from build123d import *

# Parameters (mm, degrees)
SKETCH1_R           = 2.5
SKETCH1_W           = 50
SKETCH1_H           = 22.5
BOSS_EXTRUDE1_DEPTH = 3


with BuildPart() as part:
    # Sketch1 → Boss-Extrude1 (new body)
    # profile 1 of 7: a face of its own
    with BuildSketch(Plane.XY):
        with BuildLine():
            ThreePointArc((22.5, 0), (15.909902577, 15.909902577), (0, 22.5))
            Line((0, 22.5), (-22.5, 0))
            ThreePointArc((-22.5, 0), (-22.471786645, -1.126412439), (-22.387217335, -2.25))
            ThreePointArc((-22.387217335, -2.25), (1.126412439, -22.471786645), (22.5, 0))
        make_face()
        with BuildLine():
            ThreePointArc((-7.5, 5), (-9.267766953, 9.267766953), (-5, 7.5))
            Line((-5, 7.5), (-5, 9))
            Line((-5, 9), (-2.405779746, 18.179870439))
            ThreePointArc((-2.405779746, 18.179870439), (0, 20), (2.405779746, 18.179870439))
            Line((2.405779746, 18.179870439), (5, 9))
            Line((5, 9), (5, 7.5))
            ThreePointArc((5, 7.5), (7.5, 10), (10, 7.5))
            ThreePointArc((10, 7.5), (9.267766953, 5.732233047), (7.5, 5))
            Line((7.5, 5), (9, 5))
            Line((9, 5), (18.179870439, 2.405779746))
            ThreePointArc((18.179870439, 2.405779746), (19.493699588, 1.508363998), (20, 0))
            ThreePointArc((20, 0), (19.493699588, -1.508363998), (18.179870439, -2.405779746))
            Line((18.179870439, -2.405779746), (9, -5))
            Line((9, -5), (7.5, -5))
            ThreePointArc((7.5, -5), (9.267766953, -5.732233047), (10, -7.5))
            ThreePointArc((10, -7.5), (7.5, -10), (5, -7.5))
            Line((5, -7.5), (5, -9))
            Line((5, -9), (2.405779746, -18.179870439))
            ThreePointArc((2.405779746, -18.179870439), (0, -20), (-2.405779746, -18.179870439))
            Line((-2.405779746, -18.179870439), (-5, -9))
            Line((-5, -9), (-5, -7.5))
            ThreePointArc((-5, -7.5), (-9.267766953, -9.267766953), (-7.5, -5))
            Line((-7.5, -5), (-9, -5))
            Line((-9, -5), (-18.179870439, -2.405779746))
            ThreePointArc((-18.179870439, -2.405779746), (-20, 0), (-18.179870439, 2.405779746))
            Line((-18.179870439, 2.405779746), (-9, 5))
            Line((-9, 5), (-7.5, 5))
        make_face(mode=Mode.SUBTRACT)
    # profile 2 of 7: a face of its own
    with BuildSketch(Plane.XY):
        with Locations((-7.5, 7.5)):
            Circle(SKETCH1_R)
    # profile 3 of 7: a face of its own
    with BuildSketch(Plane.XY):
        with Locations((7.5, 7.5)):
            Circle(SKETCH1_R)
    # profile 4 of 7: a face of its own
    with BuildSketch(Plane.XY):
        with Locations((7.5, -7.5)):
            Circle(SKETCH1_R)
    # profile 5 of 7: a face of its own
    with BuildSketch(Plane.XY):
        with Locations((-7.5, -7.5)):
            Circle(SKETCH1_R)
    # profile 6 of 7: a face of its own
    with BuildSketch(Plane.XY):
        Polygon((-22.5, 22.5), (0, 22.5), (-22.5, 0), align=None)
    # profile 7 of 7: a face of its own
    with BuildSketch(Plane.XY):
        with Locations((-47.5, 11.25)):
            Rectangle(SKETCH1_W, SKETCH1_H)
    extrude(amount=BOSS_EXTRUDE1_DEPTH)


solid = part.part
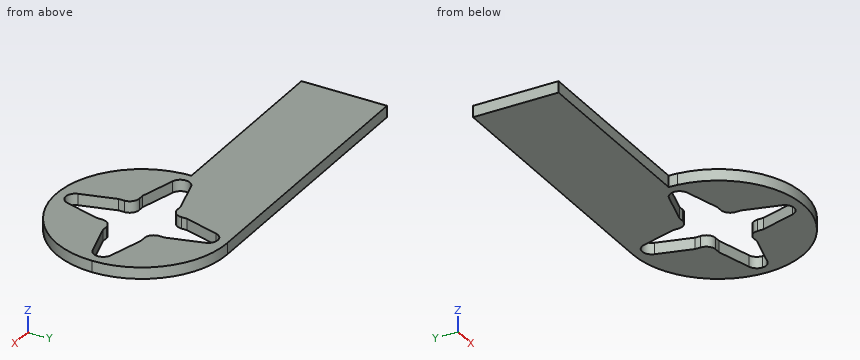
The model under review builds one solid part; all positions refer to its coordinate system, in mm. Round coordinates to 2 decimals unless told otherwise and drop trailing zeros. Loops run counter-clockwise (first coordinate to the right, second up) from the corner with the lowest first, then second, coordinate; pieces in that order, holes last. Notation, with made-up numbers: (28, -22.5) - (60, -22.5) arc R37 ccw to (60, 14.5) - close; hole circle Ø2 at (85, -39.75). An arc over 180 degrees is marked (long way). Use CSV: the item, a comma, the result in double quotes.
(1) Clearance check with flat-ended pins moving along their axes: P1, Ø0.8, axis at x = 8, z = 2, coming from the -Y side; P2, Ø1, axis at y = -15, z = 1, coming from the +X side; P3, Ø1.2, axis at y = 8, z = 2, coming from the +X side. State where each tip first meets the part, or that it passes through.
Working result:
P1,"stops at y = -21.18"
P2,"stops at x = 17.2"
P3,"stops at x = 21.25"
(2) Take a section at B-B, the plane y = -4. Give the boundary of the cut face in (x, z), plus the area to 3 significant figures.
Working result:
outline,"(-22.14, 0) - (-12.54, 0) - (-12.54, 3) - (-22.14, 3) - close; (12.54, 0) - (22.14, 0) - (22.14, 3) - (12.54, 3) - close"
area,"57.6 mm^2"
(3) Take a section at D-D, the plane x = -56.5. Give the boundary of the cut face in (y, z), plus the area to 3 significant figures.
Working result:
outline,"(0, 0) - (22.5, 0) - (22.5, 3) - (0, 3) - close"
area,"67.5 mm^2"
(4) For line 1 (Y direction, x = -41, z = 2.3); line 2 (X direction, y = 13.5, z = 2.75); line 3 (X direction, y = 7.5, z = 0.4), list the stretches that pass through material, from the lowest coordinate up.
Working result:
line 1,"y = 0 to 22.5"
line 2,"x = -72.5 to -3.73, 3.73 to 18"
line 3,"x = -72.5 to -5, 5 to 21.21"
(5) Take a section at A-A, the plane z = 2.1. Give the boundary of the cut face in (x, y), plus the area to 3 significant figures.
Working result:
outline,"(-72.5, 0) - (-22.5, 0) arc R22.5 ccw (long way) to (0, 22.5) - (-72.5, 22.5) - close; hole (-18.18, -2.41) - (-9, -5) - (-7.5, -5) arc R2.5 cw to (-5, -7.5) - (-5, -9) - (-2.41, -18.18) arc R2.5 ccw to (2.41, -18.18) - (5, -9) - (5, -7.5) arc R2.5 cw to (7.5, -5) - (9, -5) - (18.18, -2.41) arc R2.5 ccw to (18.18, 2.41) - (9, 5) - (7.5, 5) arc R2.5 cw to (5, 7.5) - (5, 9) - (2.41, 18.18) arc R2.5 ccw to (-2.41, 18.18) - (-5, 9) - (-5, 7.5) arc R2.5 cw to (-7.5, 5) - (-9, 5) - (-18.18, 2.41) arc R2.5 ccw to start"
area,"2,260 mm^2"
(6) Take a section at C-C, the plane x = 6. Give the boundary of the cut face in (y, z).
Working result:
outline,"(-21.69, 0) - (-5.5, 0) - (-5.5, 3) - (-21.69, 3) - close; (5.5, 0) - (21.69, 0) - (21.69, 3) - (5.5, 3) - close"
